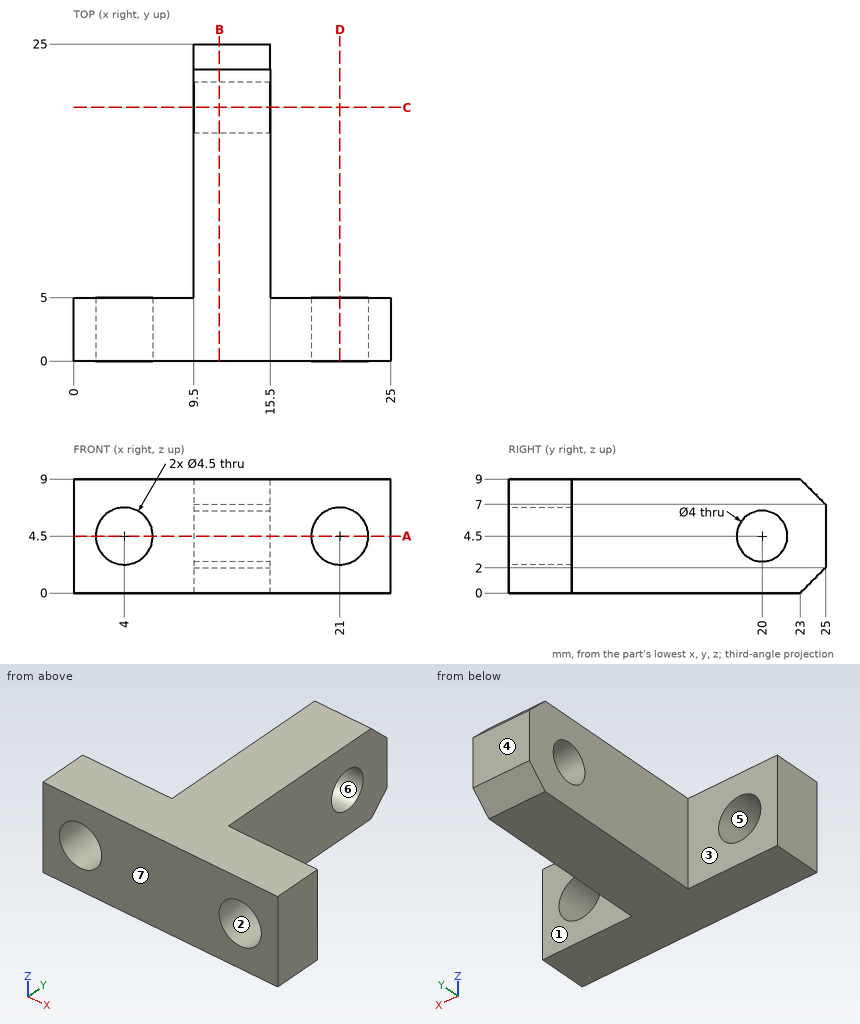
Here's the drawing with two shaded views (mm, measured from the low corner). I have some questions. A direction names the side the tool comes from. Give positions to 0.01 mm unless a question says otherwise; leave off trailing zeros. Write each loop counter-clockwise with the first axis right and the second up, starting at its lowest first coordinate (ties: lowest second). Pieces come first, ordered by that corner, then holes. Notation, with made-up numbers: (-9, 34.5) - (21, 34.5) arc R23 ccw to (21, 58.5) - close; hole circle Ø4 at (28, 61). An arc over 180 degrees is marked (long way). One line per item, written item: value. Start each with the question number.
Item 1: Imagine slicing it at A-A, the plane z = 4.5. List the corners of the cut face in (x, y) for me, and give its area (3 significant figures).
Item 2: I'm going to push flat-ended pins straight in: pin 1 (2.5 mm diameter, centred on x = 6, z = 6.5, fed in from +Y); pin 2 (5 mm diameter, centred on y = 20, z = 4.5, fed in from -X); pin 3 (1.5 mm diameter, centred on x = 16.5, y = 12.5, fed in from -Z); pin 4 (1 mm diameter, centred on y = 9.5, z = 5, fed in from +X). Where does each tip first touch, or does it pass through?
Item 3: Which directions (+Z, -Z, +X, -X, +Y, -Y) give clear straight access to the entire face, cutting with the end or side of a thin tool? Please do the marked faces 1, 2 and 3.
Item 4: Imagine slicing it at C-C, the plane y = 20. List the corners of the cut face in (x, z) for me, and give its area (3 significant figures).
Item 5: If we mould it in two halves opening along Y, with no side actions, what happens to the marked faces 4, 5, 6 and 7? For each: +Y half, -Y half, draft (parallel to the pull), parting line (faces both ways), or undercut.
Item 6: Imagine slicing it at D-D, the plane x = 21. List the corners of the cut face in (y, z) for me, and give its area (3 significant figures).
Item 7: Imagine slicing it at B-B, the plane x = 11.5. List the corners of the cut face in (y, z) for me.
Item 8: Please list where these lines run through material, in increasing order: line 1 (Z direction, x = 11.4, y = 20); line 2 (Z direction, x = 21, y = 3.4); line 3 (Y direction, x = 18.5, z = 2.5). Write a range as from..to.
Geometry says:
1. outline: (0, 0) - (1.75, 0) - (1.75, 5) - (0, 5) - close; (6.25, 0) - (18.75, 0) - (18.75, 5) - (15.5, 5) - (15.5, 18) - (9.5, 18) - (9.5, 5) - (6.25, 5) - close; (9.5, 22) - (15.5, 22) - (15.5, 25) - (9.5, 25) - close; (23.25, 0) - (25, 0) - (25, 5) - (23.25, 5) - close
1. area: 176 mm^2
2. pin 1: y = 5
2. pin 2: x = 9.5
2. pin 3: through
2. pin 4: x = 15.5
3. face 1: +Z, -Z, +X, +Y
3. face 2: +Y, -Y
3. face 3: +Z, -Z, -X, +Y
4. outline: (9.5, 0) - (15.5, 0) - (15.5, 2.5) - (9.5, 2.5) - close; (9.5, 6.5) - (15.5, 6.5) - (15.5, 9) - (9.5, 9) - close
4. area: 30.0 mm^2
5. face 4: +Y half
5. face 5: draft
5. face 6: undercut
5. face 7: -Y half
6. outline: (0, 0) - (5, 0) - (5, 2.25) - (0, 2.25) - close; (0, 6.75) - (5, 6.75) - (5, 9) - (0, 9) - close
6. area: 22.5 mm^2
7. outline: (0, 0) - (23, 0) - (25, 2) - (25, 7) - (23, 9) - (0, 9) - close; hole circle Ø4 at (20, 4.5)
8. line 1: 0..2.5, 6.5..9
8. line 2: 0..2.25, 6.75..9
8. line 3: 0..5
